Job drawing, mm, ordinate dimensions from the low corner. One solid piece. A direction names the side the tool comes from. Round coordinates to 2 decimals unless told otherwise and drop trailing zeros. Loops run counter-clockwise (first coordinate to the right, second up) from the corner with the lowest first, then second, coordinate; pieces in that order, holes last.
1) Mould opens along X. For the marked faces 1, 2 and 3 say: +X half, -X half, draft (parallel to the pull), parting line (faces both ways), or undercut.
2) Band-saw the part on A-A, the plane x = 28. Write the cut outline in (y, z) (1 decimal).
3) Band-saw the part on C-C, the plane z = 19. Write the cut outline in (x, y), then the cut area to 3 significant figures.
4) Band-saw the part on D-D, the plane z = 2.5. Write the cut outline in (x, y), then the cut area to 3 significant figures.
5) 3-axis set-ups, long thin cutter, end or side, ignore diameter. For the marked faces 4 and 5: which of +Z, -Z, +X, -X, +Y, -Y reach the whole face in a straight line?
6) Probe line 1 (Z direction, x = 18, y = 3); line 2 (Z direction, x = 12, y = 3.75); line 3 (X direction, y = 5.5, z = 20.5) (1 decimal). List the from-to ranges inside material, lowest first.
7) Drop flat-ended pins along their axis: P1, Ø8, axis at x = 6, y = 13.5, coming from the -Z side; P2, Ø5.5, axis at x = 5.5, y = 9, coming from the +Z side; P3, Ø2, axis at x = 23.5, y = 17.5, coming from the -Z side. Give the stop position or say it passes through.
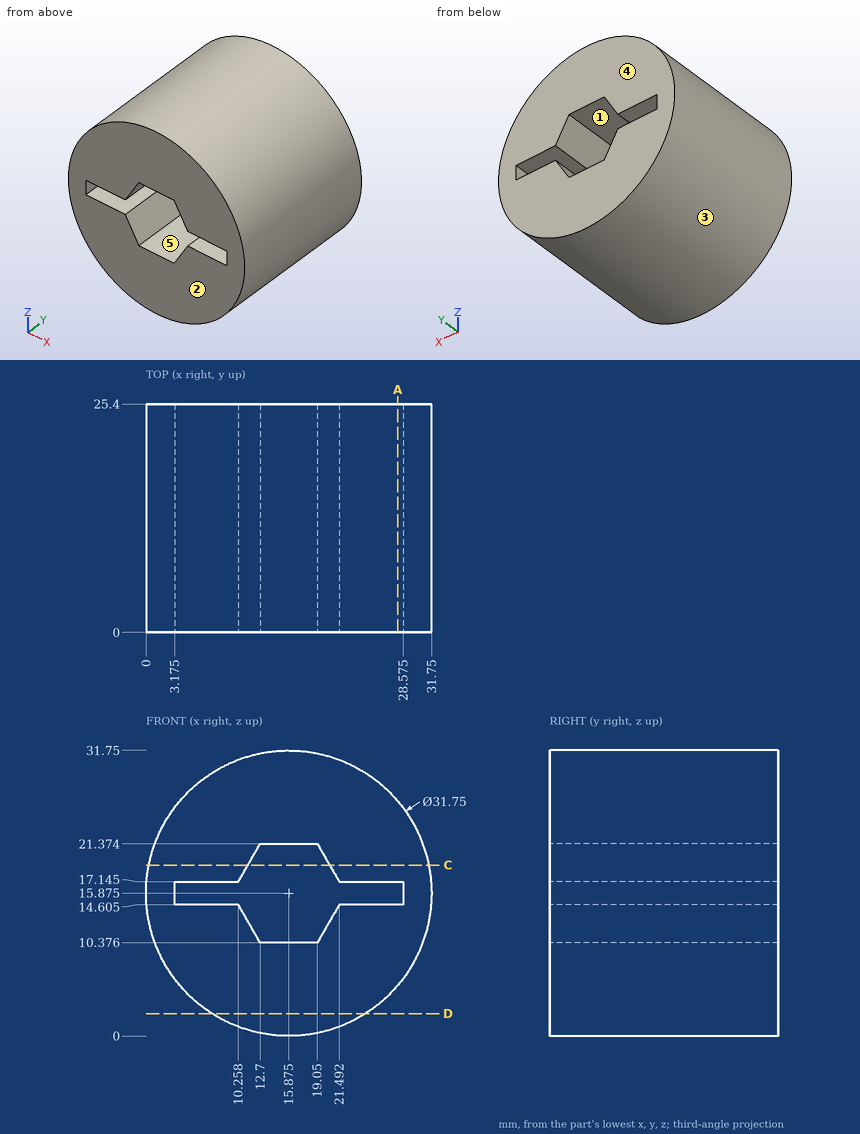
Reported:
1. face 1: undercut
1. face 2: draft
1. face 3: parting line
2. outline: (0, 5.6) - (25.4, 5.6) - (25.4, 14.6) - (0, 14.6) - close; (0, 17.1) - (25.4, 17.1) - (25.4, 26.1) - (0, 26.1) - close
3. outline: (0.31, 0) - (11.33, 0) - (11.33, 25.4) - (0.31, 25.4) - close; (20.42, 0) - (31.44, 0) - (31.44, 25.4) - (20.42, 25.4) - close
3. area: 560 mm2
4. outline: (7.32, 0) - (24.43, 0) - (24.43, 25.4) - (7.32, 25.4) - close
4. area: 434 mm2
5. face 4: +Z, -Z, +X, -X, +Y
5. face 5: +Y, -Y
6. line 1: z = 0.14 to 10.38, 21.37 to 31.61
6. line 2: z = 0.48 to 11.59, 20.16 to 31.27
6. line 3: x = 0.7 to 12.2, 19.6 to 31.1
7. P1: stops at z = 1.13
7. P2: stops at z = 29.8
7. P3: stops at z = 1.45
